from build123d import *

# Parameters (mm, degrees)
SKETCH_1_R      = 1.45
EXTRUDE_1_DEPTH = 5
SKETCH_2_R      = 1.49
EXTRUDE_2_DEPTH = 4.5
EXTRUDE_START   = 4.5
SKETCH_5_R      = 1.49
EXTRUDE_3_DEPTH = 4.5
FILLET_1_R      = 0.25


with BuildPart() as part:
    # 스케치1 → 보스-돌출1 (new body)
    with BuildSketch(Plane.XY):
        Circle(SKETCH_1_R)
    extrude(amount=EXTRUDE_1_DEPTH)

    # 스케치2 → 보스-돌출2 (add)
    with BuildSketch(Plane.XY.offset(5)):
        Circle(SKETCH_2_R)
    extrude(amount=EXTRUDE_2_DEPTH)

    # 스케치5 → 보스-돌출3 (add)
    with BuildSketch(Plane(origin=(0, 0, 0), x_dir=(-1, 0, 0), z_dir=(0, 0, -1)).offset(EXTRUDE_START)):
        with Locations(Location((0, 0, 0), (0, 0, 180))):
            Circle(SKETCH_5_R)
    extrude(amount=-EXTRUDE_3_DEPTH)

    # 필렛1
    fillet_1_edges = [part.edges().sort_by_distance(p)[0] for p in [
        (-1.49, 0, -4.5),
        (-1.49, 0, 9.5),
    ]]
    fillet(fillet_1_edges, radius=FILLET_1_R)


solid = part.part
For this review, take the finished solid that the model builds, in its own axes (mm). Round coordinates to 2 decimals unless told otherwise and drop trailing zeros. Order: outer loops, then holes, each group sorted by start corner. A loop starts at its lowest first (then second) coordinate and runs counter-clockwise, first axis right, second up. Notation, with made-up numbers: M 62.5,-29 L 73.5,-29 A19 ccw 73.5,-17 Z; hole C -18.5,19 d7. An arc over 180 degrees is marked long. Write each question's results on one line, items separated by ' | '. Start each with the question number.
1. Clearance check with flat-ended pins moving along their axes: pin 1 Ø1.5 at (y, z) = (1, 2.5) entering from -X; pin 2 Ø1.5 at (y, z) = (-0.5, 4.5) entering from +X; pin 3 Ø1 at (y, z) = (1, 0.5) entering from +X. State where each tip first meets the part, or that it passes through.
2. To check wall thickness, follow L1, parallel to X at y = 0.1, z = -3; L2, parallel to X at y = -0.6, z = 0.75. State the ranges of each line that lie inside material, in increasing order. Write a range as [from, to].
3. Draft analysis for pull direction Z (two halves, no side actions). For faces 1 (the face through (-0.194, 1.477, 7.095)), 2 (the face through (0, 0, -4.5)), 3 (the face through (-1.45, 0.06, 2.46)), state which applies: pulls with the +Z half, pulls with the -Z half, needs draft (parallel to the pull), parting line crosses it, or undercut.
4. Add section A-A (z = -2). State the section outline as (x, y) points.
5. Add section B-B (z = 3). State the section outline as (x, y) points.
Output values:
1) pin 1: x = -1.43 | pin 2: x = 1.49 | pin 3: x = 1.36
2) L1: [-1.49, 1.49] | L2: [-1.32, 1.32]
3) face 1: needs draft | face 2: pulls with the -Z half | face 3: undercut
4) outline: C 0,0 d2.98
5) outline: C 0,0 d2.9
